For this review, take the finished solid that the model builds, in its own axes (mm). Coordinates: 2 decimals unless noted, no trailing zeros. Loops run counter-clockwise (first coordinate to the right, second up) from the corner with the lowest first, then second, coordinate; pieces in that order, holes last. Notation, with made-up numbers: M 43.5,5 L 91.5,5 A25 ccw 91.5,31 Z; hole C 80.5,27.5 d6. An arc over 180 degrees is marked long. Put each result on its own line as item: value.
```python
from build123d import *

# Parameters (mm, degrees)
SKETCH1_R               = 4
SKETCH1_R_2             = 5
BOSS_EXTRUDE1_DEPTH     = 17
SKETCH1_3_R             = 4
BOSS_EXTRUDE2_DEPTH     = 49
SKETCH2_R               = 1.5
CUT_EXTRUDE1_DEPTH      = 6
CUT_EXTRUDE1_DEPTH_BACK = 6


with BuildPart() as part:
    # Sketch1 → Boss-Extrude1 (new body)
    with BuildSketch(Plane(origin=(0, 0, 0), x_dir=(1, 0, 0), z_dir=(0, 1, 0))):
        Circle(SKETCH1_R)
        Circle(SKETCH1_R_2)
        Circle(SKETCH1_R, mode=Mode.SUBTRACT)
    extrude(amount=BOSS_EXTRUDE1_DEPTH)

    # Sketch1<3> → Boss-Extrude2 (add)
    with BuildSketch(Plane(origin=(0, 0, 0), x_dir=(1, 0, 0), z_dir=(0, 1, 0))):
        Circle(SKETCH1_3_R)
    extrude(amount=BOSS_EXTRUDE2_DEPTH)

    # Sketch2 → Cut-Extrude1 (cut, two sides)
    with BuildSketch(Plane.XY) as cut_extrude1_sk:
        with Locations((0, 45)):
            Circle(SKETCH2_R)
        with Locations((0, 4)):
            Circle(SKETCH2_R)
    extrude(amount=CUT_EXTRUDE1_DEPTH, mode=Mode.SUBTRACT)
    extrude(cut_extrude1_sk.sketch, amount=-CUT_EXTRUDE1_DEPTH_BACK, mode=Mode.SUBTRACT)


solid = part.part
```
(1) Add section D-D (x = 3). Write out the cut boundary in (y, z).
Determined:
outline: M 0,-4 L 17,-4 L 17,-2.65 L 49,-2.65 L 49,2.65 L 17,2.65 L 17,4 L 0,4 Z
(2) Add section B-B (z = 1.5). Write out the cut boundary in (x, y).
Determined:
outline: M -4.77,0 L 4.77,0 L 4.77,17 L 3.71,17 L 3.71,49 L -3.71,49 L -3.71,17 L -4.77,17 Z; hole C 0,4 d3; hole C 0,45 d3
(3) Wall thickness on line 1 along Y through (x, z) = (0, -0.5); line 2 along Y through (x, z) = (-1, 0.25); line 3 along Y through (x, z) = (2, -4): over which ranges is each line inside the solid? List them lowest first. Write a range as [from, to].
Determined:
line 1: y = [0, 2.5], [5.5, 43.5], [46.5, 49]
line 2: y = [0, 2.88], [5.12, 43.88], [46.12, 49]
line 3: y = [0, 17]
(4) For pin 1 (1.8 mm diameter, centred on x = 0, y = 4, fed in from -Z); pin 2 (3.5 mm diameter, centred on x = 0, y = 45, fed in from +Z); pin 3 (1 mm diameter, centred on y = 14.5, z = -1.5, fed in from -X); pin 4 (1 mm diameter, centred on y = 34, z = -0.5, fed in from -X), all flat-tipped, find the tip position at first contact; note any pin that passes through.
Determined:
pin 1: passes through
pin 2: stops at z = 4
pin 3: stops at x = -4.9
pin 4: stops at x = -4
(5) Draft analysis for pull direction X (two halves, no side actions). For faces 1 (the cylindrical face through (-0.325, 43.536, 0.056)), 2 (the flat face through (0, 0, 0)), 3 (the cylindrical face through (-0.867, 32.776, 3.905)), state which applies: +X half, -X half, draft (parallel to the pull), parting line (faces both ways), or undercut.
Determined:
face 1: undercut
face 2: draft
face 3: parting line
(6) Add section A-A (x = 0). Write out the cut boundary in (y, z).
Determined:
outline: M 0,-5 L 2.5,-5 L 2.5,5 L 0,5 Z; M 5.5,-5 L 17,-5 L 17,-4 L 43.5,-4 L 43.5,4 L 17,4 L 17,5 L 5.5,5 Z; M 46.5,-4 L 49,-4 L 49,4 L 46.5,4 Z
(7) Add section C-C (y = 24.5). Write out the cut boundary in (x, z).
Determined:
outline: C 0,0 d8
